Can you work these out from the model? Positions are in its coordinate system, mm. Coordinates: 2 decimals unless noted, no trailing zeros. Order: outer loops, then holes, each group sorted by start corner. A loop starts at its lowest first (then second) coordinate and runs counter-clockwise, first axis right, second up. Notation, with made-up numbers: (19.5, -20.5) - (44.5, -20.5) arc R30 ccw to (44.5, 10.5) - close; hole circle Ø3 at (72.5, 83). An arc over 180 degrees is marked (long way). Use a Markdown table: item, result. Add a question column.
(1) We'd pull the mould along X, two halves only. Please class faces 1 (the flat face through (0, 31, 2)), 2 (the cylindrical face through (-54.73, 33.18, 1.61)), 3 (the flat face through (-34.44, 54.27, 1.57)): pulls with the +X half, pulls with the -X half, needs draft (parallel to the pull), parting line crosses it, or undercut.
(2) If I drill on L1, parallel to X at y = 31, z = 2.6; L2, parallel to Y at x = -62.5, z = 1.7; L3, parallel to Y at x = -53, z = 2.55, over which ranges is the centre line in solid material (lowest first)? Write a range as [from, to].
(3) I want a section at D-D (y = 12). List the corners of the cut face in (x, z) for me (3 decimals), and give its area (3 significant figures).
(4) I want a section at C-C (x = -17.5). List the corners of the cut face in (y, z) for me (3 decimals).
(5) I want a section at A-A (y = 31.75). List the corners of the cut face in (x, z) for me (3 decimals), and give its area (3 significant figures).
```python
from build123d import *

# Parameters (mm, degrees)
SALIENTE_EXTRUIR1_DEPTH = 3.175
CROQUIS2_R              = 4.7625
CORTAR_EXTRUIR1_DEPTH   = 3.175
REDONDEO1_R             = 10


with BuildPart() as part:
    # Croquis1 → Saliente-Extruir1 (new body)
    with BuildSketch(Plane.XY):
        Polygon((0, 0), (0, 63.5), (-77.274066103, 42.794476392), (-77.274066103, 20.705523608), align=None)
    extrude(amount=SALIENTE_EXTRUIR1_DEPTH)

    # Croquis2 → Cortar-Extruir1 (cut)
    with BuildSketch(Plane.XY.offset(3.175)):
        with Locations((-59.274066103, 31.75)):
            Circle(CROQUIS2_R)
    extrude(amount=-CORTAR_EXTRUIR1_DEPTH, mode=Mode.SUBTRACT)

    # Redondeo1
    redondeo1_edges = [part.edges().sort_by_distance(p)[0] for p in [
        (-77.274066103, 20.705523608, 1.5875),
        (-77.274066103, 42.794476392, 1.5875),
    ]]
    fillet(redondeo1_edges, radius=REDONDEO1_R)


solid = part.part
```
Answers follow:
| question | item | result |
|---|---|---|
| 1 | face 1 | pulls with the +X half |
| 1 | face 2 | undercut |
| 1 | face 3 | pulls with the -X half |
| 2 | L1 | x = [-77.27, -63.98], [-54.57, 0] |
| 2 | L2 | y = [16.75, 28.25], [35.25, 46.75] |
| 2 | L3 | y = [14.2, 49.3] |
| 3 | outline | (-44.785, 0) - (0, 0) - (0, 3.175) - (-44.785, 3.175) - close |
| 3 | area | 142 mm² |
| 4 | outline | (4.689, 0) - (58.811, 0) - (58.811, 3.175) - (4.689, 3.175) - close |
| 5 | outline | (-77.274, 0) - (-64.037, 0) - (-64.037, 3.175) - (-77.274, 3.175) - close; (-54.512, 0) - (0, 0) - (0, 3.175) - (-54.512, 3.175) - close |
| 5 | area | 215 mm² |
